```python
from build123d import *

# Parameters (mm, degrees)
SKETCH1_W          = 10
SKETCH1_H          = 8
SKETCH2_R          = 1.75
CUT_EXTRUDE1_DEPTH = 10
SKETCH2_3_R        = 3
SKETCH2_3_R_2      = 1.75
CUT_EXTRUDE2_DEPTH = 4


with BuildPart() as part:
    # Sketch1 → Revolve1 (revolve)
    with BuildSketch(Plane(origin=(0, 0, 0), x_dir=(0, 0, -1), z_dir=(1, 0, 0))):
        with Locations((18.485, 4)):
            Rectangle(SKETCH1_W, SKETCH1_H)
    revolve(axis=Axis((0, 0, 0), (0, 1, 0)))

    # Sketch2 → Cut-Extrude1 (cut)
    with BuildSketch(Plane(origin=(0, 8, 0), x_dir=(1, 0, 0), z_dir=(0, 1, 0))):
        with Locations((0, 18.1)):
            Circle(SKETCH2_R)
        with Locations((-15.675059808, 9.05)):
            Circle(SKETCH2_R)
        with Locations((-15.675059808, -9.05)):
            Circle(SKETCH2_R)
        with Locations((0, -18.1)):
            Circle(SKETCH2_R)
        with Locations((15.675059808, -9.05)):
            Circle(SKETCH2_R)
        with Locations((15.675059808, 9.05)):
            Circle(SKETCH2_R)
    extrude(amount=-CUT_EXTRUDE1_DEPTH, mode=Mode.SUBTRACT)

    # Sketch2_3 → Cut-Extrude2 (cut)
    with BuildSketch(Plane(origin=(0, 8, 0), x_dir=(1, 0, 0), z_dir=(0, 1, 0))):
        with Locations((-15.675059808, 9.05)):
            Circle(SKETCH2_3_R)
        with Locations((-15.675059808, 9.05)):
            Circle(SKETCH2_3_R_2, mode=Mode.SUBTRACT)
        with Locations((0, 18.1)):
            Circle(SKETCH2_3_R)
        with Locations((0, 18.1)):
            Circle(SKETCH2_3_R_2, mode=Mode.SUBTRACT)
        with Locations((15.675059808, 9.05)):
            Circle(SKETCH2_3_R)
        with Locations((15.675059808, 9.05)):
            Circle(SKETCH2_3_R_2, mode=Mode.SUBTRACT)
        with Locations((-15.675059808, -9.05)):
            Circle(SKETCH2_3_R)
        with Locations((-15.675059808, -9.05)):
            Circle(SKETCH2_3_R_2, mode=Mode.SUBTRACT)
        with Locations((0, -18.1)):
            Circle(SKETCH2_3_R)
        with Locations((0, -18.1)):
            Circle(SKETCH2_3_R_2, mode=Mode.SUBTRACT)
        with Locations((15.675059808, -9.05)):
            Circle(SKETCH2_3_R)
        with Locations((15.675059808, -9.05)):
            Circle(SKETCH2_3_R_2, mode=Mode.SUBTRACT)
    extrude(amount=-CUT_EXTRUDE2_DEPTH, mode=Mode.SUBTRACT)


solid = part.part
```
Model file for the job. Use its own axes, mm. A direction names the side the tool comes from. Round coordinates to 2 decimals unless told otherwise and drop trailing zeros. Order: outer loops, then holes, each group sorted by start corner. A loop starts at its lowest first (then second) coordinate and runs counter-clockwise, first axis right, second up. Notation, with made-up numbers: (12.25, -28.5) -> (36.25, -28.5) arc R11 cw to (36.25, -12.5) -> close; hole circle Ø3 at (20, 25). An arc over 180 degrees is marked (long way). Use one line per item in the form item = value.
Item 1: Drill centre lines: line 1 (Z direction, x = 0, y = 1.4) (3 decimals); line 2 (X direction, y = 2.5, z = 0) (3 decimals); line 3 (X direction, y = 5.6, z = -9.05). Where is each one in solid material? Low to high.
Returned:
line_1 = -23.485 to -19.85, -16.35 to -13.485, 13.485 to 16.35, 19.85 to 23.485
line_2 = -23.485 to -13.485, 13.485 to 23.485
line_3 = -21.67 to -18.68, -12.68 to -10, 10 to 12.68, 18.68 to 21.67
Item 2: Cut at C-C, the plane x = 12. Write the cut outline in (y, z), and give its area (3 significant figures).
Returned:
outline = (0, -20.19) -> (8, -20.19) -> (8, -6.15) -> (0, -6.15) -> close; (0, 6.15) -> (8, 6.15) -> (8, 20.19) -> (0, 20.19) -> close
area = 225 mm^2
Item 3: Flat gauge pins, fed straight in: pin 1 Ø5 at (x, z) = (13.5, 5.5) entering from -Y; pin 2 Ø1.8 at (x, z) = (-15, 8) entering from +Y; pin 3 Ø1 at (x, y) = (11.5, 1.5) entering from -Z; pin 4 Ø4 at (y, z) = (3, -6) entering from +X. Where does each tip first touch, or does it go through?
Returned:
pin_1 = 0
pin_2 = 4
pin_3 = -20.75
pin_4 = 23.14
Item 4: Tool access for faces 1 (the face through (13.164, 4.056, 2.923)), 2 (the face through (-14, 4, 10)): list every direction of +Z, -Z, +X, -X, +Y, -Y with a clear straight run to the whole face (end or side of a thin tool).
Returned:
face_1 = +Y, -Y
face_2 = +Y
Item 5: Cut at D-D, the plane z = 9.05. Write the cut outline in (x, y), and give its area (3 significant figures).
Returned:
outline = (-21.67, 0) -> (-17.43, 0) -> (-17.43, 4) -> (-18.68, 4) -> (-18.68, 8) -> (-21.67, 8) -> close; (-13.93, 0) -> (-10, 0) -> (-10, 8) -> (-12.68, 8) -> (-12.68, 4) -> (-13.93, 4) -> close; (10, 0) -> (13.93, 0) -> (13.93, 4) -> (12.68, 4) -> (12.68, 8) -> (10, 8) -> close; (17.43, 0) -> (21.67, 0) -> (21.67, 8) -> (18.68, 8) -> (18.68, 4) -> (17.43, 4) -> close
area = 111 mm^2
Item 6: Cut at B-B, the plane y = 5. Write the cut outline in (x, z) (3 decimals), and give its area (3 significant figures).
Returned:
outline = circle Ø46.97 at (0, 0); hole circle Ø6 at (-15.675, -9.05); hole circle Ø6 at (-15.675, 9.05); hole circle Ø26.97 at (0, 0); hole circle Ø6 at (0, -18.1); hole circle Ø6 at (0, 18.1); hole circle Ø6 at (15.675, -9.05); hole circle Ø6 at (15.675, 9.05)
area = 992 mm^2
Item 7: Pull direction X, two halves, no side cores. Call faces 3 (the face through (-17.886, 6.028, -11.078)), 4 (the face through (22.927, 4.056, 5.091)), 5 (the face through (10, 0, 10)): released by +X, released by -X, zero draft, split by the parting line, or undercut.
Returned:
face_3 = undercut
face_4 = split by the parting line
face_5 = zero draft
Item 8: Cut at A-A, the plane z = 0. Write the cut outline in (x, y) (3 decimals), and give its area (3 significant figures).
Returned:
outline = (-23.485, 0) -> (-13.485, 0) -> (-13.485, 8) -> (-23.485, 8) -> close; (13.485, 0) -> (23.485, 0) -> (23.485, 8) -> (13.485, 8) -> close
area = 160 mm^2
